Source: three-view drawing plus pictorial views. Frame: mm from the lowest corner of the part. Give positions to 0.01 mm unless a question says otherwise; leave off trailing zeros. Loops run counter-clockwise (first coordinate to the right, second up) from the corner with the lowest first, then second, coordinate; pieces in that order, holes last. Notation, with made-up numbers: M 44.25,66.25 L 71.25,66.25 A16 ccw 71.25,75.25 Z; hole C 83.25,23 d2. An arc over 180 degrees is marked long. Answer as a JSON object with one key per item and string values. Group by question number.
1) First-contact query: P1, Ø5, axis at x = 4, y = 60, coming from the +Z side (3 decimals). Flat tip, straight axial feed; report the tip coordinate or a pass-through.
2) Section query B-B on x = 16. Return loops of the section in (y, z) (3 decimals).
3) Section query D-D on x = 11. Return loops of the section in (y, z) (3 decimals).
4) Ray query, L1, parallel to Y at x = 28, z = 1.6; L2, parallel to Y at x = 2.5, z = 1.9; L3, parallel to Y at x = 16, z = 2. Return the intervals inside material, ascending.
5) Section query A-A on y = 60. Return loops of the section in (x, z) (3 decimals), plus the area to 3 significant figures.
6) Section query C-C on y = 52. Return loops of the section in (x, z) (3 decimals).
7) Draft query along Y for the marked faces 1 and 2. Return one class per face: +Y half, -Y half, draft (parallel to the pull), parting line (faces both ways), or undercut.
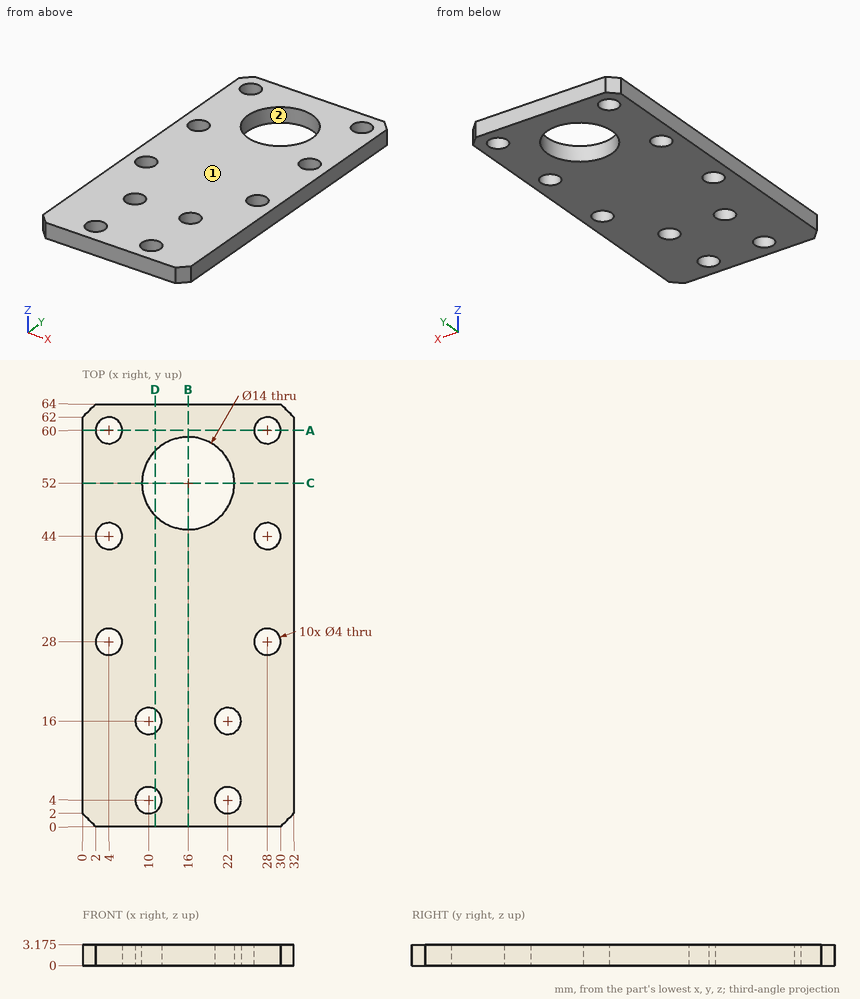
Output:
{
 "1": {"P1": "stops at z = 3.175"},
 "2": {"outline": "M 0,0 L 45,0 L 45,3.175 L 0,3.175 Z; M 59,0 L 64,0 L 64,3.175 L 59,3.175 Z"},
 "3": {"outline": "M 0,0 L 2.268,0 L 2.268,3.175 L 0,3.175 Z; M 5.732,0 L 14.268,0 L 14.268,3.175 L 5.732,3.175 Z; M 17.732,0 L 47.101,0 L 47.101,3.175 L 17.732,3.175 Z; M 56.899,0 L 64,0 L 64,3.175 L 56.899,3.175 Z"},
 "4": {"L1": "y = 0 to 26, 30 to 42, 46 to 58, 62 to 64", "L2": "y = 0 to 26.68, 29.32 to 42.68, 45.32 to 58.68, 61.32 to 64", "L3": "y = 0 to 45, 59 to 64"},
 "5": {"outline": "M 0,0 L 2,0 L 2,3.175 L 0,3.175 Z; M 6,0 L 26,0 L 26,3.175 L 6,3.175 Z; M 30,0 L 32,0 L 32,3.175 L 30,3.175 Z", "area": "76.2 mm^2"},
 "6": {"outline": "M 0,0 L 9,0 L 9,3.175 L 0,3.175 Z; M 23,0 L 32,0 L 32,3.175 L 23,3.175 Z"},
 "7": {"face 1": "draft", "face 2": "undercut"}
}
